Geometry check sheet. Reference: the model listing, model coordinates, mm. A direction names the side the tool comes from. Round coordinates to 2 decimals unless told otherwise and drop trailing zeros. Order: outer loops, then holes, each group sorted by start corner. A loop starts at its lowest first (then second) coordinate and runs counter-clockwise, first axis right, second up. Notation, with made-up numbers: (16.5, 11.25) -> (66.5, 11.25) arc R26 ccw to (66.5, 27.25) -> close; hole circle Ø9 at (28.25, 25). An arc over 180 degrees is marked (long way). Use a Markdown table: item, result. Add a question column.
Item 1: Sectioned sample at C-C, the plane x = 6.5. Record the cut outline in (y, z).
Item 2: Material ranges on probe 1 along Z at (x, y) = (0.5, 0.5); probe 2 along X at (y, z) = (-2.75, 2.5); probe 3 along X at (y, z) = (0.5, 1.5), recorded low to high. Write a range as [from, to].
Item 3: Set-up check for faces 1 (the flat face through (6, -1, -1)), 2 (the flat face through (0.453, -0.054, -4.141)), 3 (the flat face through (0.453, -0.054, 4.159)): record each of +Z, -Z, +X, -X, +Y, -Y from which the full face is reachable in a straight line by a thin tool's end or side.
Item 4: Gauge pin test, flat ends, axial feed: pin 1 Ø0.6 at (x, y) = (0.5, 0.5) entering from +Z; pin 2 Ø3 at (y, z) = (-3, -3) entering from +X; pin 3 Ø4 at (x, z) = (2.5, -0.5) entering from +Y. Record the tip position at first contact, or that the pin passes through.
Item 5: Sectioned sample at D-D, the plane z = -4. Record the cut outline in (x, y).
Item 6: Sectioned sample at B-B, the plane y = -2.5. Record the cut outline in (x, z).
Item 7: Sectioned sample at A-A, the plane z = 0. Record the cut outline in (x, y).
Item 8: Mould release check, pull along X, two halves, no side actions. Record for faces 4 (the flat face through (-0.35, 0, 0)), 5 (the flat face through (0, -2.2, 1.2)), 6 (the cylindrical face through (7, -1, 0)): pulls with the +X half, pulls with the -X half, needs draft (parallel to the pull), parting line crosses it, or undercut.
from build123d import *
from OCP.BRepFilletAPI import BRepFilletAPI_MakeChamfer

# Parameters (mm, degrees)
SKETCH1_R           = 2.35
BOSS_EXTRUDE1_DEPTH = 6
BOSS_EXTRUDE1_TAPER = 5
BOSS_EXTRUDE2_DEPTH = 0.35
SKETCH3_W           = 1.3
SKETCH3_H           = 2
BOSS_EXTRUDE3_DEPTH = 0.7
CHAMFER1_SIZE       = 0.5
CHAMFER1_SIZE2      = 1.866025404
FILLET2_R           = 0.5
FILLET3_R           = 0.25
SKETCH4_R           = 1
BOSS_EXTRUDE4_DEPTH = 8


with BuildPart() as part:
    # Sketch1 → Boss-Extrude1 (new body)
    with BuildSketch(Plane(origin=(0, 0, 0), x_dir=(0, 0, -1), z_dir=(1, 0, 0))):
        Circle(SKETCH1_R)
    extrude(amount=BOSS_EXTRUDE1_DEPTH, taper=BOSS_EXTRUDE1_TAPER)

    # Sketch2 → Boss-Extrude2 (add)
    with BuildSketch(Plane(origin=(0, 0, 0), x_dir=(0, 0, -1), z_dir=(1, 0, 0))):
        with BuildLine():
            Line((1, -4.6), (5, -4.6))
            Line((5, -4.6), (5, 2.495381949))
            Line((5, 2.495381949), (5, 2.884339454))
            ThreePointArc((5, 2.884339454), (0, 4), (-5, 2.884339454))
            Line((-5, 2.884339454), (-5, 2.495381949))
            Line((-5, 2.495381949), (-5, -4.6))
            Line((-5, -4.6), (-1, -4.6))
            Line((-1, -4.6), (-1, -3.1))
            Line((-1, -3.1), (1, -3.1))
            Line((1, -3.1), (1, -4.6))
        make_face()
    extrude(amount=-BOSS_EXTRUDE2_DEPTH)

    # Sketch3 → Boss-Extrude3 (add)
    with BuildSketch(Plane(origin=(0, 0, 0), x_dir=(0, 0, -1), z_dir=(1, 0, 0))):
        with Locations((-4.15, 0)):
            Rectangle(SKETCH3_W, SKETCH3_H)
        with Locations((4.15, 0)):
            Rectangle(SKETCH3_W, SKETCH3_H)
    extrude(amount=BOSS_EXTRUDE3_DEPTH)

    # Chamfer1: one chamfer whose edges measure the first distance from different faces: ONE call of the kernel's chamfer builder (chamfer() names one face for all edges)
    chamfer1_edges_1 = [part.edges().sort_by_distance(p)[0] for p in [
        (0.7, -1, 4.15),
    ]]
    chamfer1_side_1 = [part.faces().sort_by_distance(p)[0] for p in [
        (0.35, -1, 4.15),
    ]]
    chamfer1_edges_2 = [part.edges().sort_by_distance(p)[0] for p in [
        (0.7, -1, -4.15),
    ]]
    chamfer1_side_2 = [part.faces().sort_by_distance(p)[0] for p in [
        (0.35, -1, -4.15),
    ]]
    chamfer1 = BRepFilletAPI_MakeChamfer(part.part.solid().wrapped)
    for e in chamfer1_edges_1:
        chamfer1.Add(CHAMFER1_SIZE, CHAMFER1_SIZE2, e.wrapped, chamfer1_side_1[0].wrapped)  # the first distance lies on this face
    for e in chamfer1_edges_2:
        chamfer1.Add(CHAMFER1_SIZE, CHAMFER1_SIZE2, e.wrapped, chamfer1_side_2[0].wrapped)  # the first distance lies on this face
    add(Compound.cast(chamfer1.Shape()), mode=Mode.REPLACE)

    # Fillet2
    fillet2_edges = [part.edges().sort_by_distance(p)[0] for p in [
        (-0.175, -3.1, -1),
        (-0.175, -3.1, 1),
    ]]
    fillet(fillet2_edges, radius=FILLET2_R)

    # Fillet3
    fillet3_edges = [part.edges().sort_by_distance(p)[0] for p in [
        (-0.175, -4.6, 1),
        (-0.175, -4.6, 5),
        (-0.175, 2.884339454, 5),
        (-0.175, 2.884339454, -5),
        (-0.175, -4.6, -5),
        (-0.175, -4.6, -1),
    ]]
    fillet(fillet3_edges, radius=FILLET3_R)

    # Sketch4 → Boss-Extrude4 (add)
    with BuildSketch(Plane(origin=(0, 0, 0), x_dir=(0, 0, -1), z_dir=(1, 0, 0))):
        Circle(SKETCH4_R)
    extrude(amount=BOSS_EXTRUDE4_DEPTH)


solid = part.part
Found:
| question | item | result |
|---|---|---|
| 1 | outline | circle Ø2 at (0, 0) |
| 2 | probe 1 | z = [-4.8, -3.5], [-2.25, 2.25], [3.5, 4.8] |
| 2 | probe 2 | x = [-0.35, 0] |
| 2 | probe 3 | x = [-0.35, 6] |
| 3 | face 1 | +X |
| 3 | face 2 | -Z, +X, -Y |
| 3 | face 3 | +Z, +X, -Y |
| 4 | pin 1 | stops at z = 4.8 |
| 4 | pin 2 | stops at x = 0 |
| 4 | pin 3 | stops at y = 2.3 |
| 5 | outline | (-0.35, -4.6) -> (0, -4.6) -> (0, -1) -> (0.2, -1) -> (0.7, 0.87) -> (0.7, 1) -> (0, 1) -> (0, 3.3) -> (-0.35, 3.3) -> close |
| 6 | outline | (-0.35, -5) -> (0, -5) -> (0, 5) -> (-0.35, 5) -> close |
| 7 | outline | (-0.35, -3.1) -> (0, -3.1) -> (0, -2.35) -> (6, -1.83) -> (6, -1) -> (8, -1) -> (8, 1) -> (6, 1) -> (6, 1.83) -> (0, 2.35) -> (0, 4) -> (-0.35, 4) -> close |
| 8 | face 4 | pulls with the -X half |
| 8 | face 5 | pulls with the +X half |
| 8 | face 6 | needs draft |
